```python
from build123d import *

# Parameters (mm, degrees)
F1_DEPTH = 19.05
F2_SIZE  = 38.09999


# Not quite as in the source:
# - a fillet or chamfer is up to 0.001 mm smaller than in the source, because OpenCascade refuses the exact size


with BuildPart() as f1:
    # F0 (on Front) → F1 (new body, symmetric)
    with BuildSketch(Plane.XZ):
        Polygon((-346.5949795118, 19.05), (-406.4, -19.05), (406.4, -19.05), (406.4, 19.05), align=None)
    extrude(amount=F1_DEPTH, both=True)

    # F2 (size 38.1 in the source; OpenCascade refuses exactly that, so slightly less here)
    f2_edges = [f1.edges().sort_by_distance(p)[0] for p in [
        (406.4, 0, 19.05),
    ]]
    chamfer(f2_edges, length=F2_SIZE)


solid = f1.part
```
Can you work these out from the model? Positions are in its coordinate system, mm. Round coordinates to 2 decimals unless told otherwise and drop trailing zeros. Order: outer loops, then holes, each group sorted by start corner. A loop starts at its lowest first (then second) coordinate and runs counter-clockwise, first axis right, second up.
(1) If we section it at B-B (z = 8): Please give me the cut outline in (x, y), plus the area to 3 significant figures.
Results are:
outline: (-363.94, -19.05) - (379.35, -19.05) - (379.35, 19.05) - (-363.94, 19.05) - close
area: 28,300 mm2
(2) I'm going to push flat-ended pins straight in: pin 1 (3 mm diameter, centred on y = 13, z = 0.5, fed in from +X); pin 2 (4 mm diameter, centred on y = 14.5, z = -4.5, fed in from +X); pin 3 (12 mm diameter, centred on y = -14.5, z = 12.5, fed in from +X). Where does each tip first touch, or does it pass through?
Results are:
pin 1: stops at x = 388.35
pin 2: stops at x = 393.85
pin 3: stops at x = 380.85
(3) If I drill on L1, parallel to X at y = -1, z = -13; L2, parallel to X at y = 2, z = -14, over which ranges is the centre line in solid material (lowest first)?
Results are:
L1: x = -396.9 to 400.35
L2: x = -398.47 to 401.35
